Model file for the job. Use its own axes, mm. A direction names the side the tool comes from. Round coordinates to 2 decimals unless told otherwise and drop trailing zeros. Order: outer loops, then holes, each group sorted by start corner. A loop starts at its lowest first (then second) coordinate and runs counter-clockwise, first axis right, second up. Notation, with made-up numbers: M 23.25,65.5 L 75.25,65.5 A33 ccw 75.25,95.5 Z; hole C -34.5,40.5 d3. An arc over 180 degrees is marked long. Return JSON: item names as keys, results as strings. Group by question number.
Item 1: Probe line 1 along Y through (x, z) = (0, -7.65); line 2 along Y through (x, z) = (-2, 3.5); line 3 along X through (y, z) = (1.5, 3.25). List the from-to ranges inside material, lowest first.
Item 2: Pull direction X, two halves, no side cores. Call faces 4 (the face through (1.339, 7.945, -2.631)), 5 (the face through (-5.81, 7.49, 1.63)), 6 (the face through (5.25, 7.5, 4.3)): pulls with the +X half, pulls with the -X half, needs draft (parallel to the pull), parting line crosses it, or undercut.
Item 3: Which spindle directions (+Z, -Z, +X, -X, +Y, -Y) get a long thin tool onto all of the face, cutting with end or side? Do faces 1 (the face through (-1.75, 2.5, 6.4)), 2 (the face through (2, 5, -5)), 3 (the face through (-4.37, 1.281, 6.378)). Say none if no direction does.
Item 4: Pin check, flat tips, straight feed: pin 1 Ø5 at (x, y) = (5, 7.5) entering from +Z; pin 2 Ø1.5 at (y, z) = (5, 3.5) entering from -X; pin 3 Ø1.5 at (y, z) = (8.5, -5.5) entering from +X. Stop position of each tip, or through.
Item 5: Slice it at C-C on x = 0.25. Write the cut outline in (y, z) (3 decimals).
Item 6: Slice it at B-B on y = 2. Give the number of separate pieces and of enclosed holes in the cut face, then the cut area to 3 significant figures.
Item 7: Slice it at D-D on y = 5.5. Write the cut outline in (x, z) (3 decimals).
Item 8: Slice it at A-A on z = -1.5. Write the cut outline in (x, y), then the cut area to 3 significant figures.
from build123d import *

# Parameters (mm, degrees)
SKETCH1_W                            = 4.75
SKETCH1_H                            = 7
FILLET1_R                            = 1
SKETCH16_W                           = 16
SKETCH16_H                           = 1
CUT_EXTRUDE5_DEPTH                   = 1
CUT_EXTRUDE5_DIRECTION_2_REACH       = 18.492
CUT_EXTRUDE6_REACH                   = 15.304
SKETCH17_W                           = 3.5
SKETCH17_H                           = 5.261387212
CUT_EXTRUDE7_DEPTH                   = 18.408690359
CUT_EXTRUDE7_DEPTH_BACK              = 18.408690359
SKETCH18_R                           = 1.2
CUT_EXTRUDE10_START                  = -6
SKETCH21_R                           = 1.27
CUT_EXTRUDE10_DEPTH                  = 6
CUT_EXTRUDE11_DEPTH                  = 18.26991621
CUT_EXTRUDE11_DEPTH_BACK             = 18.26991621
SKETCH22_R                           = 1.2
CUT_EXTRUDE9_REACH                   = 20.603
CUT_EXTRUDE9_END_RADIUS              = 8
SKETCH20_R                           = 1.2
CUT_EXTRUDE12_REACH                  = 21.585
SKETCH19_R                           = 2.25
CUT_EXTRUDE13_REACH                  = 21.585
CUT_EXTRUDE13_END_RADIUS             = 8
SKETCH24_R                           = 2.25
CUT_EXTRUDE14_REACH                  = 18.492
CUT_EXTRUDE14_END_RADIUS             = 8
SKETCH25_W                           = 2.25
SKETCH25_H                           = 1
CUT_EXTRUDE14_DIRECTION_2_REACH      = 18.492
CUT_EXTRUDE14_DIRECTION_2_END_RADIUS = 8
M2_5_CLEARANCE_HOLE1_D               = 2.9
M2_5_CLEARANCE_HOLE1_DEPTH           = 8.029752102
M2_5_CLEARANCE_HOLE1_TIP             = 0.871247898
CUT_EXTRUDE15_START                  = -12
SKETCH29_W                           = 4
SKETCH29_H                           = 2.25
CUT_EXTRUDE15_DEPTH                  = 12
FILLET3_R                            = 0.25
SKETCH30_R                           = 8
CUT_EXTRUDE19_DEPTH                  = 1
BOSS_EXTRUDE1_START                  = 1
BOSS_EXTRUDE1_DEPTH                  = 1


with BuildPart() as part:
    # Sketch1 → Revolve1 (revolve)
    with BuildSketch(Plane.XY, mode=Mode.PRIVATE) as revolve1_sk:
        with Locations((5.625, 3.5)):
            Rectangle(SKETCH1_W, SKETCH1_H)
    revolve(revolve1_sk.sketch.rotate(Axis((0, 0, 0), (0, 1, 0)), 90), axis=Axis((0, 0, 0), (0, 1, 0)))

    # Sketch1<3> → Revolve2 (revolve)
    with BuildSketch(Plane.XY, mode=Mode.PRIVATE) as revolve2_sk:
        Polygon((1.27, 7), (3.25, 7), (8, 7), (8, 12), (1.27, 12), align=None)
    revolve(revolve2_sk.sketch.rotate(Axis((0, 0, 0), (0, 1, 0)), 90), axis=Axis((0, 0, 0), (0, 1, 0)))

    # Fillet1
    fillet1_edges = [part.edges().sort_by_distance(p)[0] for p in [
        (0, 12, 8),
    ]]
    fillet(fillet1_edges, radius=FILLET1_R)

    # Sketch16 → Cut-Extrude5 (cut)
    with BuildSketch(Plane.XY):
        with Locations((0, 5.5)):
            Rectangle(SKETCH16_W, SKETCH16_H)
    extrude(amount=-CUT_EXTRUDE5_DEPTH, mode=Mode.SUBTRACT)

    # Sketch16 → Cut-Extrude5 direction 2 (cut, up to next)
    with BuildSketch(Plane.XY, mode=Mode.PRIVATE) as cut_extrude5_direction_2_sk1:
        with Locations((0, 5.5)):
            Rectangle(SKETCH16_W, SKETCH16_H)
    cut_extrude5_direction_2_tool1 = extrude(cut_extrude5_direction_2_sk1.sketch, amount=CUT_EXTRUDE5_DIRECTION_2_REACH, mode=Mode.PRIVATE) & part.part
    add(cut_extrude5_direction_2_tool1.solids().sort_by_distance((0, 5.5, 0))[0], mode=Mode.SUBTRACT)

    # Sketch17 → Cut-Extrude6 (cut, up to next)
    with BuildSketch(Plane(origin=(0, 5, 0), x_dir=(1, 0, 0), z_dir=(0, 1, 0)), mode=Mode.PRIVATE) as cut_extrude6_sk1:
        with Locations((0, -5.369306394)):
            Rectangle(SKETCH17_W, SKETCH17_H)
    cut_extrude6_tool1 = extrude(cut_extrude6_sk1.sketch, amount=-CUT_EXTRUDE6_REACH, mode=Mode.PRIVATE) & part.part
    add(cut_extrude6_tool1.solids().sort_by_distance((0, 5, 5.369306))[0], mode=Mode.SUBTRACT)

    # Sketch18 → Cut-Extrude7 (cut, two sides: drawn at the far end of the back side and taken through both)
    with BuildSketch(Plane.ZY.offset(-1.75).offset(-CUT_EXTRUDE7_DEPTH_BACK)):
        with Locations((4.772430143, 2.5)):
            Circle(SKETCH18_R)
    extrude(amount=CUT_EXTRUDE7_DEPTH + CUT_EXTRUDE7_DEPTH_BACK, mode=Mode.SUBTRACT)

    # Sketch21 → Cut-Extrude10 (cut)
    with BuildSketch(Plane(origin=(0, 12, 0), x_dir=(1, 0, 0), z_dir=(0, 1, 0)).offset(CUT_EXTRUDE10_START)):
        Circle(SKETCH21_R)
        Polygon((-1.5, -1.9), (-1.5, -11.891029443), (1.5, -11.891029443), (1.5, -1.9), (0.896046874, -1.9), (0.896046874, -0.9), (-0.896046874, -0.9), (-0.896046874, -1.9), align=None)
    extrude(amount=CUT_EXTRUDE10_DEPTH, mode=Mode.SUBTRACT)

    # Sketch22 → Cut-Extrude11 (cut, two sides: drawn at the far end of the back side and taken through both)
    with BuildSketch(Plane(origin=(-1.5, 0, 0), x_dir=(0, 0, -1), z_dir=(1, 0, 0)).offset(-CUT_EXTRUDE11_DEPTH_BACK)):
        with Locations((-3.358116823, 8.5)):
            Circle(SKETCH22_R)
    extrude(amount=CUT_EXTRUDE11_DEPTH + CUT_EXTRUDE11_DEPTH_BACK, mode=Mode.SUBTRACT)

    # Cut-Extrude9: up to this cylinder (the profile starts inside it)
    cut_extrude9_end = Plane(origin=(0, 5.9847245, 0), z_dir=(0, -1, 0)) * Cylinder(CUT_EXTRUDE9_END_RADIUS, 65.175449, mode=Mode.PRIVATE)
    # Sketch20 → Cut-Extrude9 (cut, up to the surface)
    with BuildSketch(Plane(origin=(-3.75, 0, 0), x_dir=(0, 0, -1), z_dir=(1, 0, 0)), mode=Mode.PRIVATE) as cut_extrude9_sk1:
        Polygon((-2.463029066, 2.5), (-3.617729604, 4.5), (-5.927130681, 4.5), (-7.08183122, 2.5), (-5.927130681, 0.5), (-3.617729604, 0.5), align=None)
    cut_extrude9_tool1 = extrude(cut_extrude9_sk1.sketch, amount=-CUT_EXTRUDE9_REACH, mode=Mode.PRIVATE) & cut_extrude9_end
    add(cut_extrude9_tool1.solids().sort_by_distance((-3.75, 2.5, 4.77243))[0], mode=Mode.SUBTRACT)
    # Sketch20 → Cut-Extrude9 (cut, up to the surface)
    with BuildSketch(Plane(origin=(-3.75, 0, 0), x_dir=(0, 0, -1), z_dir=(1, 0, 0)), mode=Mode.PRIVATE) as cut_extrude9_sk2:
        Polygon((-1.048715746, 8.5), (-2.203416284, 10.5), (-4.512817361, 10.5), (-5.6675179, 8.5), (-4.512817361, 6.5), (-2.203416284, 6.5), align=None)
        with Locations((-3.358116823, 8.5)):
            Circle(SKETCH20_R, mode=Mode.SUBTRACT)
    cut_extrude9_tool2 = extrude(cut_extrude9_sk2.sketch, amount=-CUT_EXTRUDE9_REACH, mode=Mode.PRIVATE) & cut_extrude9_end
    add(cut_extrude9_tool2.solids().sort_by_distance((-3.75, 9.469449, 1.678981))[0], mode=Mode.SUBTRACT)

    # Sketch19 → Cut-Extrude12 (cut, up to next)
    with BuildSketch(Plane.ZY.offset(-5.25), mode=Mode.PRIVATE) as cut_extrude12_sk1:
        with Locations((4.772430143, 2.5)):
            Circle(SKETCH19_R)
    cut_extrude12_tool1 = extrude(cut_extrude12_sk1.sketch, amount=-CUT_EXTRUDE12_REACH, mode=Mode.PRIVATE) & part.part
    add(cut_extrude12_tool1.solids().sort_by_distance((5.25, 2.5, 4.77243))[0], mode=Mode.SUBTRACT)

    # Cut-Extrude13: up to this cylinder (the profile starts inside it)
    cut_extrude13_end = Plane(origin=(0, 8.5, 0), z_dir=(0, -1, 0)) * Cylinder(CUT_EXTRUDE13_END_RADIUS, 60.17, mode=Mode.PRIVATE)
    # Sketch24 → Cut-Extrude13 (cut, up to the surface)
    with BuildSketch(Plane.ZY.offset(-5.25), mode=Mode.PRIVATE) as cut_extrude13_sk1:
        with Locations((3.358116823, 8.5)):
            Circle(SKETCH24_R)
    cut_extrude13_tool1 = extrude(cut_extrude13_sk1.sketch, amount=-CUT_EXTRUDE13_REACH, mode=Mode.PRIVATE) & cut_extrude13_end
    add(cut_extrude13_tool1.solids().sort_by_distance((5.25, 8.5, 3.358117))[0], mode=Mode.SUBTRACT)

    # Cut-Extrude14: up to this cylinder (the profile starts inside it)
    cut_extrude14_end = Plane(origin=(0, 5.5, 0), z_dir=(0, -1, 0)) * Cylinder(CUT_EXTRUDE14_END_RADIUS, 53.984, mode=Mode.PRIVATE)
    # Sketch25 → Cut-Extrude14 (cut, up to the surface)
    with BuildSketch(Plane.ZY, mode=Mode.PRIVATE) as cut_extrude14_sk1:
        with Locations((-2.125, 5.5)):
            Rectangle(SKETCH25_W, SKETCH25_H)
    cut_extrude14_tool1 = extrude(cut_extrude14_sk1.sketch, amount=-CUT_EXTRUDE14_REACH, mode=Mode.PRIVATE) & cut_extrude14_end
    add(cut_extrude14_tool1.solids().sort_by_distance((0, 5.5, -2.125))[0], mode=Mode.SUBTRACT)

    # Cut-Extrude14 direction 2: up to this cylinder (the profile starts inside it)
    cut_extrude14_direction_2_end = Plane(origin=(0, 5.5, 0), z_dir=(0, -1, 0)) * Cylinder(CUT_EXTRUDE14_DIRECTION_2_END_RADIUS, 53.984, mode=Mode.PRIVATE)
    # Sketch25 → Cut-Extrude14 direction 2 (cut, up to the surface)
    with BuildSketch(Plane.ZY, mode=Mode.PRIVATE) as cut_extrude14_direction_2_sk1:
        with Locations((-2.125, 5.5)):
            Rectangle(SKETCH25_W, SKETCH25_H)
    cut_extrude14_direction_2_tool1 = extrude(cut_extrude14_direction_2_sk1.sketch, amount=CUT_EXTRUDE14_DIRECTION_2_REACH, mode=Mode.PRIVATE) & cut_extrude14_direction_2_end
    add(cut_extrude14_direction_2_tool1.solids().sort_by_distance((0, 5.5, -2.125))[0], mode=Mode.SUBTRACT)

    # M2.5 Clearance Hole1
    with Locations(Plane(origin=(0, 0, -8), x_dir=(-1, 0, 0), z_dir=(0, 0, -1))):
        with Locations((0, 8.5), (0, 2.5)):
            Hole(M2_5_CLEARANCE_HOLE1_D / 2, depth=M2_5_CLEARANCE_HOLE1_DEPTH)
            with Locations((0, 0, -(M2_5_CLEARANCE_HOLE1_DEPTH + M2_5_CLEARANCE_HOLE1_TIP / 2))):  # 118° drill point
                Cone(0, M2_5_CLEARANCE_HOLE1_D / 2, M2_5_CLEARANCE_HOLE1_TIP, mode=Mode.SUBTRACT)

    # Sketch29 → Cut-Extrude15 (cut)
    with BuildSketch(Plane(origin=(0, 12, 0), x_dir=(1, 0, 0), z_dir=(0, 1, 0)).offset(CUT_EXTRUDE15_START)):
        with Locations((0, 5.5)):
            Rectangle(SKETCH29_W, SKETCH29_H)
    extrude(amount=CUT_EXTRUDE15_DEPTH, mode=Mode.SUBTRACT)

    # Fillet3
    fillet3_edges = [part.edges().sort_by_distance(p)[0] for p in [
        (0.896046874, 9.5, 1.9),
        (-0.896046874, 9.5, 1.9),
    ]]
    fillet(fillet3_edges, radius=FILLET3_R)

    # Sketch30 → Cut-Extrude19 (cut)
    with BuildSketch(Plane(origin=(0, 12, 0), x_dir=(1, 0, 0), z_dir=(0, 1, 0))):
        Circle(SKETCH30_R)
    extrude(amount=-CUT_EXTRUDE19_DEPTH, mode=Mode.SUBTRACT)

    # Sketch31 → Boss-Extrude1 (add)
    with BuildSketch(Plane.XZ.offset(-7).offset(BOSS_EXTRUDE1_START)):
        with BuildLine():
            Line((-0.896046874, 0.9), (-0.896046874, 1.65))
            ThreePointArc((-0.896046874, 1.65), (-0.969270178, 1.826776695), (-1.146046874, 1.9))
            Line((-1.146046874, 1.9), (-1.5, 1.9))
            Line((-1.5, 1.9), (-1.5, 2.883140649))
            ThreePointArc((-1.5, 2.883140649), (0, -3.25), (1.5, 2.883140649))
            Line((1.5, 2.883140649), (1.5, 1.9))
            Line((1.5, 1.9), (1.146046874, 1.9))
            ThreePointArc((1.146046874, 1.9), (0.969270178, 1.826776695), (0.896046874, 1.65))
            Line((0.896046874, 1.65), (0.896046874, 0.9))
            ThreePointArc((0.896046874, 0.9), (0, -1.27), (-0.896046874, 0.9))
        make_face()
    extrude(amount=-BOSS_EXTRUDE1_DEPTH)


solid = part.part
Output values:
{
 "1": {"line 1": "0 to 1.05, 3.95 to 7.05, 9.95 to 11", "line 2": "0 to 5, 6 to 7.31, 9.69 to 11", "line 3": "-3.75 to -1.75, 1.75 to 5.25"},
 "2": {"face 4": "undercut", "face 5": "needs draft", "face 6": "pulls with the +X half"},
 "3": {"face 1": "+Z, -Y", "face 2": "+Y, -Y", "face 3": "-X"},
 "4": {"pin 1": "z = 7.6", "pin 2": "x = -7.51", "pin 3": "x = 6.44"},
 "5": {"outline": "M 0,-7.996 L 1.072,-7.996 L 1.072,-6.625 L 0,-6.625 Z; M 0,-4.375 L 1.072,-4.375 L 1.072,-3.24 L 0,-3.24 Z; M 3.928,-7.996 L 7.072,-7.996 L 7.072,-6.625 L 3.928,-6.625 Z; M 3.928,-4.375 L 7.072,-4.375 L 7.072,-1.245 L 6,-1.245 L 6,-3.25 L 5,-3.25 L 5,-3.24 L 3.928,-3.24 Z; M 9.928,-7.996 L 11,-7.996 L 11,-6.625 L 9.928,-6.625 Z; M 9.928,-4.375 L 11,-4.375 L 11,-1.245 L 9.928,-1.245 Z"},
 "6": {"separate pieces": "4", "enclosed holes": "0", "area": "108 mm²"},
 "7": {"outline": "M -7.31,-3.25 A8 ccw 7.31,-3.25 Z; hole M -2,-6.625 L 2,-6.625 L 2,-4.375 L -2,-4.375 Z"},
 "8": {"outline": "M -7.86,0 L -2.88,0 L -2.88,5 L -7.86,5 Z; M -7.86,6 L 7.86,6 L 7.86,11 L -7.86,11 Z; M 2.88,0 L 7.86,0 L 7.86,5 L 2.88,5 Z; hole C 0,8.5 d2.9", "area": "122 mm²"}
}
